Build history of the part. All positions in model axes, mm. A direction names the side the tool comes from. Give positions to 0.01 mm unless a question says otherwise; leave off trailing zeros. Write each loop counter-clockwise with the first axis right and the second up, starting at its lowest first coordinate (ties: lowest second). Pieces come first, ordered by that corner, then holes. Notation, with made-up numbers: (69, 74.25) -> (123, 74.25) arc R17 ccw to (123, 81.25) -> close; hole circle Ø6 at (-18.75, 52). An arc over 180 degrees is marked (long way). One line per question, with ' | ' between items. Start each with the question number.
(1) Pull direction Z, two halves, no side cores. Call faces 4 (the flat face through (-56, -33, 6)), 5 (the flat face through (-10.58, 68.61, 13.44)), 6 (the cylindrical face through (13.305, 67.71, 7.479)): released by +Z, released by -Z, zero draft, split by the parting line, or undercut.
(2) Band-saw the part on C-C, the plane z = 2.75. Count the separate pieces of the cut face and the enclosed holes in it, and give its area (3 significant figures).
(3) Band-saw the part on A-A, the plane y = 39. Give the cut face in (x, z).
(4) Tool access for faces 1 (the flat face through (-67.76, -29.57, 7.48)), 2 (the flat face through (-18.92, 74.52, 13.4)), 3 (the flat face through (-8.75, 84, 9)): list every direction of +Z, -Z, +X, -X, +Y, -Y with a clear straight run to the whole face (end or side of a thin tool).
(5) Band-saw the part on B-B, the plane x = -43. Give the cut face in (y, z).
(6) Pin check, flat tips, straight feed: P1, Ø3, axis at y = 97.5, z = 9, coming from the -X side; P2, Ø12, axis at y = 31.5, z = 18.5, coming from the -X side; P3, Ø0.9, axis at x = -15.5, z = 22.5, coming from the +Y side. Stop position of each tip, or through.
(7) Drill centre lines: probe 1 along Y at (x, z) = (56.5, 6.75); probe 2 along X at (y, z) = (-26, 14.25); probe 3 along Y at (x, z) = (42.5, 5.5). Where is each one in solid material? Low to high. Write a range as from..to.
from build123d import *

# Parameters (mm, degrees)
PAD_DEPTH             = 24
POCKET_DEPTH          = 3
SKETCH002_W           = 70
SKETCH002_H           = 18.5
POCKET001_DEPTH       = 18
POLARPATTERN_COUNT    = 3
POCKET002_DEPTH       = 6
CHAMFER_SIZE          = 8
FILLET_R              = 13
FILLET001_R           = 11
CHAMFER001_SIZE       = 16.1
FILLET002_R           = 11
FILLET003_R           = 12
POCKET003_DEPTH       = 6
POCKET004_DEPTH       = 18
POCKET005_DEPTH       = 21.001
SKETCH007_W           = 15.5
SKETCH007_H           = 15
POCKET006_DEPTH       = 5
SKETCH010_W           = 13.6
SKETCH010_H           = 9
POCKET009_DEPTH       = 15.5
POCKET010_DEPTH       = 3
SKETCH012_R           = 1.85
SKETCH012_R_2         = 0.99
POCKET011_DEPTH       = 498.0492855781
POLARPATTERN001_COUNT = 3
POCKET012_DEPTH       = 12
POCKET013_DEPTH       = 3
POCKET014_DEPTH       = 3


with BuildPart() as part:
    # Sketch → Pad (new body)
    with BuildSketch(Plane.XY):
        Polygon((0, 112.2094915052), (-97.1762701892, -56.1047457526), (97.1762701892, -56.1047457526), align=None)
        Polygon((0, 62.2094915052), (-53.875, -31.1047457526), (53.875, -31.1047457526), align=None, mode=Mode.SUBTRACT)
    extrude(amount=PAD_DEPTH)

    # Sketch001 (on Face8 of Pad) → Pocket (cut)
    with BuildSketch(Plane.XY.offset(24)):
        Polygon((0, 98.2094915052), (-85.0519145362, -49.1047457526), (85.0519145362, -49.1047457526), align=None)
        Polygon((0, 76.2094915052), (-65.999355653, -38.1047457526), (65.999355653, -38.1047457526), align=None, mode=Mode.SUBTRACT)
    extrude(amount=-POCKET_DEPTH, mode=Mode.SUBTRACT)

    # Sketch002 (on Face4 of Pocket) → Pocket001 (cut)
    with BuildSketch(Plane(origin=(0, 0, 0), x_dir=(1, 0, 0), z_dir=(0, 0, -1))):
        with Locations((0, 43.6047457526)):
            Rectangle(SKETCH002_W, SKETCH002_H)
    pocket001 = extrude(amount=-POCKET001_DEPTH, mode=Mode.SUBTRACT)

    # PolarPattern: Pocket001 ×3 about axis
    polarpattern_axis = Axis((0, 0, 0), (0, 0, -1))
    for i in range(1, POLARPATTERN_COUNT):
        add(pocket001.rotate(polarpattern_axis, i * 360 / POLARPATTERN_COUNT), mode=Mode.SUBTRACT)

    # Sketch003 (on Face4 of PolarPattern) → Pocket002 (cut)
    with BuildSketch(Plane(origin=(0, 0, 0), x_dir=(1, 0, 0), z_dir=(0, 0, -1))):
        Polygon((0, -100.2094915052), (86.7839653438, 50.1047457526), (-86.7839653438, 50.1047457526), align=None)
        Polygon((0, -74.2094915052), (64.2673048454, 37.1047457526), (-64.2673048454, 37.1047457526), align=None, mode=Mode.SUBTRACT)
    extrude(amount=-POCKET002_DEPTH, mode=Mode.SUBTRACT)

    # Chamfer
    chamfer_edges = [part.edges().sort_by_distance(p)[0] for p in [
        (-53.875, -31.104746, 12),
        (53.875, -31.104746, 12),
        (0, 62.209492, 12),
    ]]
    chamfer(chamfer_edges, length=CHAMFER_SIZE)

    # Fillet
    fillet_edges = [part.edges().sort_by_distance(p)[0] for p in [
        (0, 100.209492, 3),
        (-86.783965, -50.104746, 3),
        (86.783965, -50.104746, 3),
    ]]
    fillet(fillet_edges, radius=FILLET_R)

    # Fillet001
    fillet001_edges = [part.edges().sort_by_distance(p)[0] for p in [
        (0, 74.209492, 3),
        (64.267305, -37.104746, 3),
        (-64.267305, -37.104746, 3),
    ]]
    fillet(fillet001_edges, radius=FILLET001_R)

    # Chamfer001
    chamfer001_edges = [part.edges().sort_by_distance(p)[0] for p in [
        (97.17627, -56.104746, 12),
        (0, 112.209492, 12),
        (-97.17627, -56.104746, 12),
    ]]
    chamfer(chamfer001_edges, length=CHAMFER001_SIZE)

    # Fillet002
    fillet002_edges = [part.edges().sort_by_distance(p)[0] for p in [
        (0, 98.209492, 22.5),
        (-85.051915, -49.104746, 22.5),
        (85.051915, -49.104746, 22.5),
    ]]
    fillet(fillet002_edges, radius=FILLET002_R)

    # Fillet003
    fillet003_edges = [part.edges().sort_by_distance(p)[0] for p in [
        (65.999356, -38.104746, 22.5),
        (0, 76.209492, 22.5),
        (-65.999356, -38.104746, 22.5),
    ]]
    fillet(fillet003_edges, radius=FILLET003_R)

    # Sketch004 (on Face60 of Fillet003) → Pocket003 (cut)
    with BuildSketch(Plane(origin=(0, 0, 6), x_dir=(1, 0, 0), z_dir=(0, 0, -1))):
        Polygon((-8.75, -72.1664825043), (8.75, -72.1664825043), (8.75, -94.7664825043), (4, -94.7664825043), (4, -98.2664825043), (-4, -98.2664825043), (-4, -94.7664825043), (-8.75, -94.7664825043), align=None)
    extrude(amount=-POCKET003_DEPTH, mode=Mode.SUBTRACT)

    # Sketch005 (on Face29 of Pocket003) → Pocket004 (cut)
    with BuildSketch(Plane(origin=(0, 0, 0), x_dir=(1, 0, 0), z_dir=(0, 0, -1))):
        Polygon((46.1715988394, 38.9547457526), (68.6882593378, 51.9547457526), (79.3382593378, 33.508404652), (56.8215988394, 20.508404652), align=None)
    extrude(amount=-POCKET004_DEPTH, mode=Mode.SUBTRACT)

    # Sketch006 (on Face1 of Pocket004) → Pocket005 (cut, through all)
    with BuildSketch(Plane.XY.offset(21)):
        with BuildLine():
            ThreePointArc((1.5, 85.0404521425), (0, 86.5404521425), (-1.5, 85.0404521425))
            Line((-1.5, 85.0404521425), (-1.5, 66.0404521425))
            ThreePointArc((-1.5, 66.0404521425), (0, 64.5404521425), (1.5, 66.0404521425))
            Line((1.5, 85.0404521425), (1.5, 66.0404521425))
        make_face()
    extrude(amount=-POCKET005_DEPTH, mode=Mode.SUBTRACT)

    # Sketch007 (on Face24 of Pocket005) → Pocket006 (cut)
    with BuildSketch(Plane(origin=(-48.5881350946, 28.0523728763, 0), x_dir=(-0.5, -0.8660254038, 0), z_dir=(-0.8660254038, 0.5, 0))):
        with Locations((-47.3262701892, 13.5)):
            Rectangle(SKETCH007_W, SKETCH007_H)
    extrude(amount=-POCKET006_DEPTH, mode=Mode.SUBTRACT)

    # Sketch010 (on Face79 of Pocket006) → Pocket009 (cut)
    with BuildSketch(Plane(origin=(-44.2580080757, 25.5523728763, 0), x_dir=(-0.5, -0.8660254038, 0), z_dir=(-0.8660254038, 0.5, 0))):
        with Locations((-47.3262701892, 13.5)):
            Rectangle(SKETCH010_W, SKETCH010_H)
    extrude(amount=-POCKET009_DEPTH, mode=Mode.SUBTRACT)

    # Sketch011 (on Face21 of Pocket009) → Pocket010 (cut)
    with BuildSketch(Plane(origin=(0, 0, 6), x_dir=(1, 0, 0), z_dir=(0, 0, -1))):
        Polygon((-21.0413798427, -59.7570681827), (-11.6817654684, -54.3532923042), (-6.658482036, -63.0538744299), (-16.0180964103, -68.4576503084), align=None)
    extrude(amount=-POCKET010_DEPTH, mode=Mode.SUBTRACT)

    # Sketch012 (on Face54 of Pocket010) → Pocket011 (cut, through all)
    with BuildSketch(Plane(origin=(0, 0, 0), x_dir=(1, 0, 0), z_dir=(0, 0, -1))):
        with Locations((-13.5, -82.7032108255)):
            Circle(SKETCH012_R)
        with Locations((13.5, -82.7032108255)):
            Circle(SKETCH012_R)
        with Locations((-6.25, -96.5164825043)):
            Circle(SKETCH012_R_2)
        with Locations((6.25, -96.5164825043)):
            Circle(SKETCH012_R_2)
        with Locations((-27.2463245869, -59.0174730012)):
            Circle(SKETCH012_R_2)
        with Locations((-47.1862074814, -27.2405827309)):
            Circle(SKETCH012_R_2)
        with Locations((-64.7337931796, 5.9127272486)):
            Circle(SKETCH012_R_2)
        with Locations((-10.791841915, -49.5174730012)):
            Circle(SKETCH012_R_2)
        with Locations((-28.3394276132, -16.3641630217)):
            Circle(SKETCH012_R_2)
        with Locations((-48.2793105078, 15.4127272487)):
            Circle(SKETCH012_R_2)
    pocket011 = extrude(amount=-POCKET011_DEPTH, mode=Mode.SUBTRACT)

    # PolarPattern001: Pocket011 ×3 about axis
    polarpattern001_axis = Axis((0, 0, 0), (0, 0, -1))
    for i in range(1, POLARPATTERN001_COUNT):
        add(pocket011.rotate(polarpattern001_axis, i * 360 / POLARPATTERN001_COUNT), mode=Mode.SUBTRACT)

    # Sketch013 (on Face132 of PolarPattern001) → Pocket012 (cut)
    with BuildSketch(Plane(origin=(0, 0, 6), x_dir=(1, 0, 0), z_dir=(0, 0, -1))):
        Polygon((58.553649647, 21.508404652), (63.3167893678, 24.258404652), (66.3167893678, 19.0622522293), (61.553649647, 16.3122522293), align=None)
    extrude(amount=-POCKET012_DEPTH, mode=Mode.SUBTRACT)

    # Sketch014 (on Face127 of Pocket012) → Pocket013 (cut)
    with BuildSketch(Plane(origin=(0, 0, 6), x_dir=(1, 0, 0), z_dir=(0, 0, -1))):
        Polygon((-74.3478338252, 33.3748379063), (-65.8478338252, 48.0972697706), (-52.8574527684, 40.5972697706), (-61.3574527684, 25.8748379063), align=None)
    extrude(amount=-POCKET013_DEPTH, mode=Mode.SUBTRACT)

    # Sketch015 (on Face21 of Pocket013) → Pocket014 (cut)
    with BuildSketch(Plane(origin=(0, 0, 6), x_dir=(1, 0, 0), z_dir=(0, 0, -1))):
        with BuildLine():
            ThreePointArc((-8.75, -63.0538744299), (-13.3063040372, -67.6101784671), (-8.75, -72.1664825043))
            Line((-8.75, -72.1664825043), (8.75, -72.1664825043))
            ThreePointArc((8.75, -72.1664825043), (13.3063040372, -67.6101784671), (8.75, -63.0538744299))
            Line((-8.75, -63.0538744299), (8.75, -63.0538744299))
        make_face()
    extrude(amount=-POCKET014_DEPTH, mode=Mode.SUBTRACT)


solid = part.part
Results:
1) face 4: released by -Z | face 5: undercut | face 6: zero draft
2) separate pieces: 2 | enclosed holes: 32 | area: 3,930 mm²
3) outline: (-42.27, 0) -> (-38.51, 0) -> (-38.51, 18) -> (-17.15, 18) -> (-17.15, 0) -> (-13.4, 0) -> (-13.4, 24) -> (-21.48, 24) -> (-21.48, 21) -> (-34.18, 21) -> (-34.18, 24) -> (-42.27, 24) -> close; (13.4, 0) -> (17.15, 0) -> (17.15, 18) -> (38.51, 18) -> (38.51, 0) -> (42.27, 0) -> (42.27, 24) -> (34.18, 24) -> (34.18, 21) -> (21.48, 21) -> (21.48, 24) -> (13.4, 24) -> close
4) face 1: -Z | face 2: -X | face 3: none
5) outline: (-56.1, 0) -> (-50.1, 0) -> (-50.1, 6) -> (-37.1, 6) -> (-37.1, 0) -> (-31.1, 0) -> (-31.1, 24) -> (-38.1, 24) -> (-38.1, 21) -> (-49.1, 21) -> (-49.1, 24) -> (-56.1, 24) -> close; (-12.27, 0) -> (-5.77, 0) -> (-5.77, 18) -> (31.23, 18) -> (31.23, 0) -> (37.73, 0) -> (37.73, 24) -> (23.73, 24) -> (23.73, 21) -> (1.73, 21) -> (1.73, 24) -> (-12.27, 24) -> close
6) P1: stops at x = -9.36 | P2: stops at x = -50.06 | P3: stops at y = 86.14
7) probe 1: y = -56.1..-44.92, -21.07..-7.79, 7.85..14.35 | probe 2: x = -79.8..-48.82, 48.82..53.65, 66.33..79.8 | probe 3: y = -56.1..-50.1, -37.1..-31.1, -11.4..-4.9, 32.1..38.6
